from build123d import *

# Parameters (mm, degrees)
SKETCH1_R           = 45
BOSS_EXTRUDE1_DEPTH = 60
RIB8_REACH          = 89.464
SKETCH4_WALL_W      = 192.619578006
SKETCH4_WALL_H      = 3
RIB9_REACH          = 89.464
SKETCH5_WALL_W      = 188.67722245
SKETCH5_WALL_H      = 3
CIRPATTERN1_COUNT   = 8
SKETCH6_W           = 6
SKETCH6_H           = 12
CUT_EXTRUDE1_DEPTH  = 30
CUT_EXTRUDE2_DEPTH  = 18
CHAMFER1_SIZE       = 0.8
CHAMFER2_SIZE       = 6
SKETCH10_R          = 2
CUT_EXTRUDE3_DEPTH  = 100.904954832
SKETCH11_R          = 2.5
BOSS_EXTRUDE2_DEPTH = 5
SKETCH12_R          = 1.5
CUT_EXTRUDE4_DEPTH  = 5
SKETCH13_R          = 1


with BuildPart() as part:
    # Sketch1 → Boss-Extrude1 (new body)
    with BuildSketch(Plane.XY):
        Circle(SKETCH1_R)
    extrude(amount=BOSS_EXTRUDE1_DEPTH)

    # Sketch3 → Cut-Revolve1 (revolve, cut)
    with BuildSketch(Plane(origin=(0, 0, 0), x_dir=(0, 0, -1), z_dir=(1, 0, 0))):
        Polygon((0, 27.5), (0, 0), (-60, 0), (-60, 5.5), (-2, 5.5), (-2, 27.5), align=None)
        Polygon((-5, 45), (-5, 25), (-55, 25), (-55, 35), (-60, 35), (-60, 45), align=None)
    revolve(axis=Axis((0, 0, 0), (0, 0, 1)), mode=Mode.SUBTRACT)

    # Sketch4 wall → Rib8 (add, up to next)
    with BuildSketch(Plane(origin=(0, 31.426666031, 9.5), x_dir=(0, -0.819152044296, 0.573576436341), z_dir=(0, -0.573576436341, -0.819152044296)), mode=Mode.PRIVATE) as rib8_sk1:
        Rectangle(SKETCH4_WALL_W, SKETCH4_WALL_H)
    rib8_tool1 = extrude(rib8_sk1.sketch, amount=RIB8_REACH, mode=Mode.PRIVATE) - part.part
    rib8 = rib8_tool1.solids().sort_by_distance((0, 31.426666031, 9.5))[0]
    add(rib8)

    # Sketch5 wall → Rib9 (add, up to next)
    with BuildSketch(Plane(origin=(0, 28.775948341, 50.5), x_dir=(0, -0.642787609707, -0.766044443102), z_dir=(0, 0.766044443102, -0.642787609707)), mode=Mode.PRIVATE) as rib9_sk1:
        Rectangle(SKETCH5_WALL_W, SKETCH5_WALL_H)
    rib9_tool1 = extrude(rib9_sk1.sketch, amount=-RIB9_REACH, mode=Mode.PRIVATE) - part.part
    rib9 = rib9_tool1.solids().sort_by_distance((0, 28.775948341, 50.5))[0]
    add(rib9)

    # CirPattern1: Rib8, Rib9 ×8 about axis
    cirpattern1_axis = Axis((0, 0, 0), (0, 0, 1))
    add([rib8.rotate(cirpattern1_axis, i * 360 / CIRPATTERN1_COUNT) for i in range(1, CIRPATTERN1_COUNT)])
    add([rib9.rotate(cirpattern1_axis, i * 360 / CIRPATTERN1_COUNT) for i in range(1, CIRPATTERN1_COUNT)])

    # Sketch6 → Cut-Extrude1 (cut, symmetric)
    with BuildSketch(Plane(origin=(0, 0, 0), x_dir=(0, 0, -1), z_dir=(1, 0, 0))):
        with Locations((-18, 19)):
            Rectangle(SKETCH6_W, SKETCH6_H)
        with Locations((-42, 19)):
            Rectangle(SKETCH6_W, SKETCH6_H)
        with Locations((-42, -19)):
            Rectangle(SKETCH6_W, SKETCH6_H)
        with Locations((-18, -19)):
            Rectangle(SKETCH6_W, SKETCH6_H)
    extrude(amount=CUT_EXTRUDE1_DEPTH, both=True, mode=Mode.SUBTRACT)

    # Sketch8 → Cut-Extrude2 (cut)
    with BuildSketch(Plane(origin=(0, 0, 21), x_dir=(-1, 0, 0), z_dir=(0, 0, -1))):
        Polygon((-11, 13), (-11, 21), (11, 21), (11, 13), (26.229477205, 13), (26.229477205, 31.577824801), (-25.591324377, 31.577824801), (-25.591324377, 13), align=None)
        Polygon((-25.591324377, -13), (-11, -13), (-11, -21), (11, -21), (11, -13), (26.229477205, -13), (26.229477205, -31.577824801), (-25.591324377, -31.577824801), align=None)
    extrude(amount=-CUT_EXTRUDE2_DEPTH, mode=Mode.SUBTRACT)

    # Chamfer1
    chamfer1_edges = [part.edges().sort_by_distance(p)[0] for p in [
        (-12.247448714, 21.794494718, 15),
        (12.247448714, 21.794494718, 45),
        (0, -25, 45),
        (0, -25, 15),
    ]]
    chamfer(chamfer1_edges, length=CHAMFER1_SIZE)

    # Chamfer2
    chamfer2_edges = [part.edges().sort_by_distance(p)[0] for p in [
        (11, 17, 21),
        (-11, 17, 21),
        (-11, 17, 39),
        (11, 17, 39),
        (11, -17, 39),
        (-11, -17, 39),
        (-11, -17, 21),
        (11, -17, 21),
    ]]
    chamfer(chamfer2_edges, length=CHAMFER2_SIZE)

    # Sketch10 → Cut-Extrude3 (cut, through all)
    with BuildSketch(Plane.XZ.offset(21)):
        with Locations(Location((-8.5, 30, 0), (0, 0, 270))):
            Circle(SKETCH10_R)
        with Locations(Location((8.5, 30, 0), (0, 0, 270))):
            Circle(SKETCH10_R)
    extrude(amount=-CUT_EXTRUDE3_DEPTH, mode=Mode.SUBTRACT)

    # Sketch11 → Boss-Extrude2 (add)
    with BuildSketch(Plane(origin=(0, 0, 0), x_dir=(-1, 0, 0), z_dir=(0, 0, -1))):
        with Locations((0, 45)):
            Circle(SKETCH11_R)
        with Locations((26.450336353, 36.405764747)):
            Circle(SKETCH11_R)
        with Locations((42.797543233, 13.905764747)):
            Circle(SKETCH11_R)
        with Locations((42.797543233, -13.905764747)):
            Circle(SKETCH11_R)
        with Locations((26.450336353, -36.405764747)):
            Circle(SKETCH11_R)
        with Locations((0, -45)):
            Circle(SKETCH11_R)
        with Locations((-26.450336353, -36.405764747)):
            Circle(SKETCH11_R)
        with Locations((-42.797543233, -13.905764747)):
            Circle(SKETCH11_R)
        with Locations((-42.797543233, 13.905764747)):
            Circle(SKETCH11_R)
        with Locations((-26.450336353, 36.405764747)):
            Circle(SKETCH11_R)
    extrude(amount=-BOSS_EXTRUDE2_DEPTH)

    # Sketch12 → Cut-Extrude4 (cut)
    with BuildSketch(Plane(origin=(0, 0, 0), x_dir=(-1, 0, 0), z_dir=(0, 0, -1))):
        with Locations((0, 45)):
            Circle(SKETCH12_R)
        with Locations((26.450336353, 36.405764747)):
            Circle(SKETCH12_R)
        with Locations((42.797543233, 13.905764747)):
            Circle(SKETCH12_R)
        with Locations((42.797543233, -13.905764747)):
            Circle(SKETCH12_R)
        with Locations((26.450336353, -36.405764747)):
            Circle(SKETCH12_R)
        with Locations((0, -45)):
            Circle(SKETCH12_R)
        with Locations((-26.450336353, -36.405764747)):
            Circle(SKETCH12_R)
        with Locations((-42.797543233, -13.905764747)):
            Circle(SKETCH12_R)
        with Locations((-42.797543233, 13.905764747)):
            Circle(SKETCH12_R)
        with Locations((-26.450336353, 36.405764747)):
            Circle(SKETCH12_R)
    extrude(amount=-CUT_EXTRUDE4_DEPTH, mode=Mode.SUBTRACT)

    # Sketch13 → Cut-Revolve2 (revolve, cut)
    with BuildSketch(Plane(origin=(0, 0, 0), x_dir=(1, 0, 0), z_dir=(0, 1, 0)), mode=Mode.PRIVATE) as cut_revolve2_sk:
        with Locations((35, -57.5)):
            Circle(SKETCH13_R)
    revolve(cut_revolve2_sk.sketch.rotate(Axis((0, 0, 0), (0, 0, 1)), 90), axis=Axis((0, 0, 0), (0, 0, 1)), mode=Mode.SUBTRACT)


solid = part.part
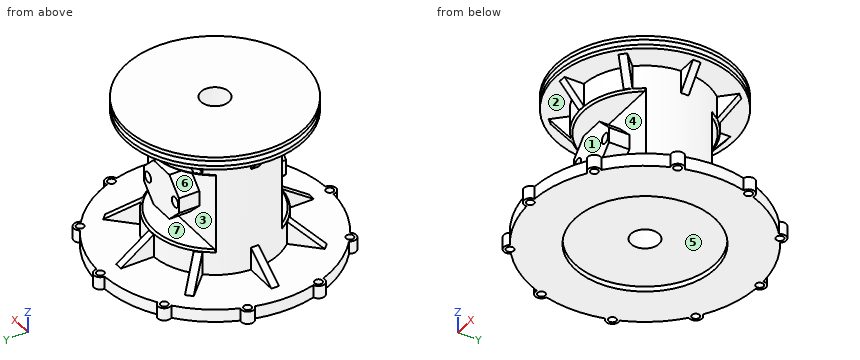
Part model, mm, in its own coordinate system. Face numbers are marked on the shaded views. A direction names the side the tool comes from. Coordinates: 2 decimals unless noted, no trailing zeros. Order: outer loops, then holes, each group sorted by start corner. A loop starts at its lowest first (then second) coordinate and runs counter-clockwise, first axis right, second up. Notation, with made-up numbers: M -18.75,86 L 40.25,86 A20 ccw 40.25,91 Z; hole C -40,49.25 d3. An arc over 180 degrees is marked long. Use a Markdown table: item, result.
(1) Cut at A-A on z = 30. Write the cut outline in (x, y).
A:
| item | result |
|---|---|
| outline | M -21.35,-13 L -11,-13 L -11,-21 L -10.5,-21 L -10.5,21 L -11,21 L -11,13 L -21.35,13 A25 ccw Z; M -6.5,-21 L 6.5,-21 L 6.5,21 L -6.5,21 Z; M 10.5,-21 L 11,-21 L 11,-13 L 21.35,-13 A25 ccw 21.35,13 L 11,13 L 11,21 L 10.5,21 Z; hole C 0,0 d11 |
(2) Tool access for the marked faces 1, 2, 3 and 4: list every direction of +Z, -Z, +X, -X, +Y, -Y with a clear straight run to the whole face (end or side of a thin tool).
A:
| item | result |
|---|---|
| face 1 | +X, -X, -Y |
| face 2 | none |
| face 3 | +Y |
| face 4 | -Y |
(3) Probe L1, parallel to Y at x = 0, z = 3.85; L2, parallel to Z at x = 20, y = 17.5; L3, parallel to Z at x = -23, y = 20.5. List the from-to ranges inside material, lowest first.
A:
| item | result |
|---|---|
| L1 | y = -47.5 to -46.5, -43.5 to -5.5, 5.5 to 43.5, 46.5 to 47.5 |
| L2 | z = 2 to 5, 55 to 60 |
| L3 | z = 0 to 5, 55 to 60 |
(4) Flat gauge pins, fed straight in: pin 1 (6.5 mm diameter, centred on y = -18.5, z = 28.5, fed in from +X); pin 2 (3 mm diameter, centred on x = -8.5, z = 30, fed in from +Y); pin 3 (1.5 mm diameter, centred on y = 3.5, z = 20, fed in from +X); pin 4 (1.5 mm diameter, centred on y = 12.5, z = 28.5, fed in from +X). Where does each tip first touch, or does it go through?
A:
| item | result |
|---|---|
| pin 1 | stops at x = 11 |
| pin 2 | passes through |
| pin 3 | stops at x = 24.85 |
| pin 4 | stops at x = 22.07 |
(5) Cut at B-B on y = 0. State how many separate pieces and enclosed holes the cut face has, then the cut area to 3 significant figures.
A:
| item | result |
|---|---|
| separate pieces | 2 |
| enclosed holes | 2 |
| area | 2,710 mm^2 |
(6) Pull direction X, two halves, no side cores. Call the marked faces 5, 6 and 7: released by +X, released by -X, zero draft, split by the parting line, or undercut.
A:
| item | result |
|---|---|
| face 5 | undercut |
| face 6 | released by -X |
| face 7 | zero draft |
